Geometry check sheet. Reference: the model listing, model coordinates, mm. A direction names the side the tool comes from. Give positions to 0.01 mm unless a question says otherwise; leave off trailing zeros. Loops run counter-clockwise (first coordinate to the right, second up) from the corner with the lowest first, then second, coordinate; pieces in that order, holes last.
1. Cross-section at B-B, the plane z = 30. State how many separate pieces and enclosed holes the cut face has, plus the area to 3 significant figures.
2. Release check for a two-part mould opening along Z. For faces 1 (the flat face through (52, 59, 59)), 2 (the cylindrical face through (61, 88, 30)), 3 (the flat face through (37, 2, 1)) record: +Z half, -Z half, draft (parallel to the pull), parting line (faces both ways), or undercut.
3. Go/stop test with flat-tipped pins: pin 1 Ø9.5 at (y, z) = (85, 30) entering from -X; pin 2 Ø15.5 at (x, z) = (12, 37.5) entering from +Y. Record where each tip stops, or that it passes through.
4. Cross-section at A-A, the plane y = 60. Record the cut outline in (x, z), plus the area to 3 significant figures.
5. Cross-section at C-C, the plane y = 35. Record the cut outline in (x, z).
6. Tool access check on faces 4 (the flat face through (19, 44, 58)), 5 (the flat face through (68, 56.6, 30)), 6 (the flat face through (18, 42, 1)), 7 (the flat face through (10, 69, 58)), 8 (the flat face through (10, 70, 30)). Record the directions out of +Z, -Z, +X, -X, +Y, -Y that give a thin tool (end or side, any length) a straight path to the whole face; none if there is none.
7. Material ranges on L1, parallel to X at y = 45, z = 5.5; L2, parallel to Z at x = 63.5, y = 35; L3, parallel to Y at x = 7, z = 16, recorded low to high.
8. Cross-section at D-D, the plane x = 7. Record the cut outline in (y, z), plus the area to 3 significant figures.
from build123d import *

# Parameters (mm, degrees)
PAD_DEPTH       = 60
POCKET_DEPTH    = 60.001
SKETCH002_R     = 3
POCKET001_DEPTH = 20.001
CHAMFER_SIZE    = 2
CHAMFER001_SIZE = 2
CHAMFER002_SIZE = 3
CHAMFER003_SIZE = 3
SKETCH003_R     = 5
POCKET002_DEPTH = 20


with BuildPart() as part:
    # Sketch → Pad (new body)
    with BuildSketch(Plane.XY):
        Polygon((0, 70), (20, 70), (20, 20), (50, 20), (50, 100), (70, 100), (70, 0), (0, 0), align=None)
    extrude(amount=PAD_DEPTH)

    # Sketch001 (on DatumPlane) → Pocket (cut, through all)
    with BuildSketch(Plane.XY.offset(60)):
        with BuildLine():
            ThreePointArc((67.267666, 63.389448), (63.602639, 60.133937), (67, 56.6))
            Line((67, 56.6), (70, 56.6))
            Line((70, 63.389448), (70, 56.6))
            Line((67.267666, 63.389448), (70, 63.389448))
        make_face()
    extrude(amount=-POCKET_DEPTH, mode=Mode.SUBTRACT)

    # Sketch002 (on Face14 of Pocket) → Pocket001 (cut, through all)
    with BuildSketch(Plane(origin=(50, 0, 0), x_dir=(0, -1, 0), z_dir=(-1, 0, 0))):
        with Locations((-85, 30)):
            Circle(SKETCH002_R)
        with Locations((-35, 30)):
            Circle(SKETCH002_R)
    extrude(amount=-POCKET001_DEPTH, mode=Mode.SUBTRACT)

    # Chamfer
    chamfer_edges = [part.edges().sort_by_distance(p)[0] for p in [
        (50, 88, 30),
    ]]
    chamfer(chamfer_edges, length=CHAMFER_SIZE)

    # Chamfer001
    chamfer001_edges = [part.edges().sort_by_distance(p)[0] for p in [
        (50, 38, 30),
    ]]
    chamfer(chamfer001_edges, length=CHAMFER001_SIZE)

    # Chamfer002
    chamfer002_edges = [part.edges().sort_by_distance(p)[0] for p in [
        (50, 100, 30),
        (50, 60, 0),
        (50, 60, 60),
    ]]
    chamfer(chamfer002_edges, length=CHAMFER002_SIZE)

    # Chamfer003
    chamfer003_edges = [part.edges().sort_by_distance(p)[0] for p in [
        (0, 35, 60),
        (0, 0, 30),
        (0, 35, 0),
        (0, 70, 30),
        (35, 0, 60),
        (35, 0, 0),
        (20, 45, 60),
        (10, 70, 60),
        (35, 20, 0),
        (20, 45, 0),
        (10, 70, 0),
        (20, 70, 30),
        (61.5, 100, 0),
        (61.5, 100, 60),
    ]]
    chamfer(chamfer003_edges, length=CHAMFER003_SIZE)

    # Sketch003 (on DatumPlane) → Pocket002 (cut)
    with BuildSketch(Plane(origin=(0, 0, 0), x_dir=(0, -1, 0), z_dir=(-1, 0, 0))):
        with Locations((-35, 30)):
            Circle(SKETCH003_R)
    extrude(amount=-POCKET002_DEPTH, mode=Mode.SUBTRACT)


solid = part.part
Result:
1. separate pieces: 4
1. enclosed holes: 0
1. area: 3,500 mm2
2. face 1: +Z half
2. face 2: undercut
2. face 3: -Z half
3. pin 1: stops at x = 50.25
3. pin 2: stops at y = 70
4. outline: (0, 3) - (3, 0) - (17, 0) - (20, 3) - (20, 57) - (17, 60) - (3, 60) - (0, 57) - close; (50, 3) - (53, 0) - (63.6, 0) - (63.6, 60) - (53, 60) - (50, 57) - close
4. area: 1,990 mm2
5. outline: (0, 3) - (3, 0) - (17, 0) - (20, 3) - (20, 25) - (0, 25) - close; (0, 35) - (20, 35) - (20, 57) - (17, 60) - (3, 60) - (0, 57) - close; (50, 3) - (53, 0) - (70, 0) - (70, 27) - (52, 27) - (50, 25) - close; (50, 35) - (52, 33) - (70, 33) - (70, 60) - (53, 60) - (50, 57) - close
6. face 4: +Z, +Y
6. face 5: +Z, -Z, +X
6. face 6: -Z, +Y
6. face 7: +Z, -X, +Y
6. face 8: +Z, -Z, -X, +Y
7. L1: x = 0 to 20, 50 to 70
7. L2: z = 0 to 27, 33 to 60
7. L3: y = 0 to 70
8. outline: (0, 3) - (3, 0) - (67, 0) - (70, 3) - (70, 57) - (67, 60) - (3, 60) - (0, 57) - close; hole circle Ø10 at (35, 30)
8. area: 4,100 mm2
